from build123d import *

# Parameters (mm, degrees)
F0_R          = 6.35
F0_R_2        = 203.2
F1_DEPTH      = 53.975
F2_DEPTH      = 104.775
F2_DEPTH_BACK = 50.8


with BuildPart() as f1:
    # F0 (on Front) → F1 (new body)
    with BuildSketch(Plane.XZ):
        Circle(F0_R)
        Circle(F0_R_2)
        Circle(F0_R, mode=Mode.SUBTRACT)
    extrude(amount=F1_DEPTH)

    # F0 (on Front) → F2 (join, two sides)
    with BuildSketch(Plane.XZ) as f2_sk:
        Circle(F0_R)
    extrude(amount=F2_DEPTH)
    extrude(f2_sk.sketch, amount=-F2_DEPTH_BACK)


solid = f1.part
Model file for the job. Use its own axes, mm. A direction names the side the tool comes from. Give positions to 0.01 mm unless a question says otherwise; leave off trailing zeros. Order: outer loops, then holes, each group sorted by start corner. A loop starts at its lowest first (then second) coordinate and runs counter-clockwise, first axis right, second up. Notation, with made-up numbers: (-21, -15) -> (-2, -15) arc R14 cw to (-2, -3) -> close; hole circle Ø4 at (57.25, 62.25). An arc over 180 degrees is marked (long way). Use CSV: the item, a comma, the result in double quotes.
1. Drill centre lines: line 1 along Z through (x, y) = (3, -10); line 2 along Y through (x, z) = (93.5, 20) (3 decimals); line 3 along X through (y, z) = (-43, -168.5). Where is each one in solid material? Low to high. Write a range as from..to.
Outcome:
line 1,"-203.18..203.18"
line 2,"-53.975..0"
line 3,"-113.57..113.57"
2. 3-axis set-ups, long thin cutter, end or side, ignore diameter. For faces 1 (the cylindrical face through (-1.38, -79.02, -6.2)), 2 (the flat face through (0, -104.775, 0)), 3 (the cylindrical face through (-1.38, 25.04, -6.2)): which of +Z, -Z, +X, -X, +Y, -Y reach the whole face in a straight line?
Outcome:
face 1,"-Y"
face 2,"+Z, -Z, +X, -X, -Y"
face 3,"+Y"
3. Band-saw the part on D-D, the plane x = -106. Give the cut face in (y, z) (3 decimals), then the cut area to 3 significant figures.
Outcome:
outline,"(-53.975, -173.362) -> (0, -173.362) -> (0, 173.362) -> (-53.975, 173.362) -> close"
area,"18,700 mm²"
4. Band-saw the part on A-A, the plane x = 0. Give the cut face in (y, z) (3 decimals), then the cut area to 3 significant figures.
Outcome:
outline,"(-104.775, -6.35) -> (-53.975, -6.35) -> (-53.975, -203.2) -> (0, -203.2) -> (0, -6.35) -> (50.8, -6.35) -> (50.8, 6.35) -> (0, 6.35) -> (0, 203.2) -> (-53.975, 203.2) -> (-53.975, 6.35) -> (-104.775, 6.35) -> close"
area,"23,200 mm²"
5. Band-saw the part on B-B, the plane z = 0. Give the cut face in (x, y) (3 decimals).
Outcome:
outline,"(-203.2, -53.975) -> (-6.35, -53.975) -> (-6.35, -104.775) -> (6.35, -104.775) -> (6.35, -53.975) -> (203.2, -53.975) -> (203.2, 0) -> (6.35, 0) -> (6.35, 50.8) -> (-6.35, 50.8) -> (-6.35, 0) -> (-203.2, 0) -> close"
6. Band-saw the part on C-C, the plane y = -83.5. Give the cut face in (x, z), then the cut area to 3 significant figures.
Outcome:
outline,"circle Ø12.7 at (0, 0)"
area,"127 mm²"
7. Drop flat-ended pins along their axis: pin 1 (1.5 mm diameter, centred on x = 26.5, y = -44.5, fed in from -Z); pin 2 (6 mm diameter, centred on x = -53.5, z = -35, fed in from -Y) (3 decimals); pin 3 (1 mm diameter, centred on x = -133, y = -21, fed in from +Z). Give the stop position or say it passes through.
Outcome:
pin 1,"z = -201.56"
pin 2,"y = -53.975"
pin 3,"z = 154.06"
